```python
from build123d import *

# Parameters (mm, degrees)
BOSS_EXTRUDE1_DEPTH      = 12.7
BOSS_EXTRUDE1_DRAFT      = -1
SKETCH8_W                = 66.675
SKETCH8_H                = 1.5875
CUT_EXTRUDE1_DEPTH       = 139.494635157
CUT_EXTRUDE1_DEPTH_BACK  = 139.494635157
CUT_EXTRUDE3_REACH       = 227.639
CUT_EXTRUDE3_END_RADIUS  = 19.05
SKETCH9_R                = 3.175
BOSS_EXTRUDE2_REACH      = 228.521
BOSS_EXTRUDE2_END_RADIUS = 19.05
BOSS_EXTRUDE2_DRAFT      = 1


with BuildPart() as part:
    # Sketch2 → Boss-Extrude1 (with draft: the straight prism first)
    with BuildSketch(Plane(origin=(0, 0, 0), x_dir=(1, 0, 0), z_dir=(0, 1, 0))):
        with BuildLine():
            Line((-113.50625, 58.7375), (-113.50625, -58.7375))
            ThreePointArc((-113.50625, -58.7375), (-94.45625, -77.7875), (-75.40625, -58.7375))
            Line((-75.40625, -58.7375), (-75.40625, -30.1625))
            Line((-75.40625, -30.1625), (75.40625, -30.1625))
            Line((75.40625, -30.1625), (75.40625, -58.7375))
            ThreePointArc((75.40625, -58.7375), (94.45625, -77.7875), (113.50625, -58.7375))
            Line((113.50625, -58.7375), (113.50625, 58.7375))
            ThreePointArc((113.50625, 58.7375), (94.45625, 77.7875), (75.40625, 58.7375))
            Line((75.40625, 58.7375), (75.40625, 30.1625))
            Line((75.40625, 30.1625), (-75.40625, 30.1625))
            Line((-75.40625, 30.1625), (-75.40625, 58.7375))
            ThreePointArc((-75.40625, 58.7375), (-94.45625, 77.7875), (-113.50625, 58.7375))
        make_face()
        with BuildLine():
            ThreePointArc((-88.9, -63.5), (-94.45625, -69.05625), (-100.0125, -63.5))
            Line((-100.0125, -63.5), (-100.0125, -53.975))
            ThreePointArc((-100.0125, -53.975), (-94.45625, -48.41875), (-88.9, -53.975))
            Line((-88.9, -53.975), (-88.9, -63.5))
        make_face(mode=Mode.SUBTRACT)
        with BuildLine():
            Line((-100.0125, 53.975), (-100.0125, 63.5))
            ThreePointArc((-100.0125, 63.5), (-94.45625, 69.05625), (-88.9, 63.5))
            Line((-88.9, 63.5), (-88.9, 53.975))
            ThreePointArc((-88.9, 53.975), (-94.45625, 48.41875), (-100.0125, 53.975))
        make_face(mode=Mode.SUBTRACT)
        with BuildLine():
            Line((100.0125, 63.5), (100.0125, 53.975))
            ThreePointArc((100.0125, 53.975), (94.45625, 48.41875), (88.9, 53.975))
            Line((88.9, 53.975), (88.9, 63.5))
            ThreePointArc((88.9, 63.5), (94.45625, 69.05625), (100.0125, 63.5))
        make_face(mode=Mode.SUBTRACT)
        with BuildLine():
            Line((100.0125, -53.975), (100.0125, -63.5))
            ThreePointArc((100.0125, -63.5), (94.45625, -69.05625), (88.9, -63.5))
            Line((88.9, -63.5), (88.9, -53.975))
            ThreePointArc((88.9, -53.975), (94.45625, -48.41875), (100.0125, -53.975))
        make_face(mode=Mode.SUBTRACT)
    extrude(amount=BOSS_EXTRUDE1_DEPTH)
    # Boss-Extrude1: the draft: its side faces are tilted about the plane it starts from
    boss_extrude1_sides = [part.faces().sort_by_distance(p)[0] for p in [
        (-113.50625, 6.35, 0),
        (-94.45625, 6.35, 77.7875),
        (-75.40625, 6.35, 44.45),
        (0, 6.35, 30.1625),
        (75.40625, 6.35, 44.45),
        (94.45625, 6.35, 77.7875),
        (113.50625, 6.35, 0),
        (94.45625, 6.35, -77.7875),
        (75.40625, 6.35, -44.45),
        (0, 6.35, -30.1625),
        (-75.40625, 6.35, -44.45),
        (-94.45625, 6.35, -77.7875),
        (-94.45625, 6.35, 48.41875),
        (-88.9, 6.35, 58.7375),
        (-94.45625, 6.35, 69.05625),
        (-100.0125, 6.35, 58.7375),
        (-100.0125, 6.35, -58.7375),
        (-94.45625, 6.35, -69.05625),
        (-88.9, 6.35, -58.7375),
        (-94.45625, 6.35, -48.41875),
        (100.0125, 6.35, -58.7375),
        (94.45625, 6.35, -48.41875),
        (88.9, 6.35, -58.7375),
        (94.45625, 6.35, -69.05625),
        (100.0125, 6.35, 58.7375),
        (94.45625, 6.35, 69.05625),
        (88.9, 6.35, 58.7375),
        (94.45625, 6.35, 48.41875),
    ]]
    draft(boss_extrude1_sides, Plane(origin=(0, 0, 0), x_dir=(1, 0, 0), z_dir=(0, 1, 0)), BOSS_EXTRUDE1_DRAFT)

    # Sketch8 → Cut-Extrude1 (cut, two sides)
    with BuildSketch(Plane.XY) as cut_extrude1_sk:
        with Locations((-33.3375, 11.90625)):
            Rectangle(SKETCH8_W, SKETCH8_H)
        with Locations((33.3375, 11.90625)):
            Rectangle(SKETCH8_W, SKETCH8_H)
    extrude(amount=CUT_EXTRUDE1_DEPTH, mode=Mode.SUBTRACT)
    extrude(cut_extrude1_sk.sketch, amount=-CUT_EXTRUDE1_DEPTH_BACK, mode=Mode.SUBTRACT)



with BuildPart() as body_2:
    # Sketch5 → Revolve2 (revolve)
    with BuildSketch(Plane.XY.offset(9.525), mode=Mode.PRIVATE) as revolve2_sk:
        with BuildLine():
            Line((141.509179325, -122.2375), (141.509179325, -128.5748))
            Line((141.509179325, -128.5748), (136.746679325, -128.5748))
            Line((136.746679325, -128.5748), (136.746679325, -126.20625))
            Line((136.746679325, -126.20625), (82.771679325, -126.20625))
            Line((82.771679325, -126.20625), (82.771679325, -128.5748))
            Line((82.771679325, -128.5748), (78.009179325, -128.5748))
            Line((78.009179325, -128.5748), (78.009179325, -122.2375))
            ThreePointArc((78.009179325, -122.2375), (78.474147309, -121.114967985), (79.596679325, -120.65))
            Line((79.596679325, -120.65), (139.921679325, -120.65))
            ThreePointArc((139.921679325, -120.65), (141.04421134, -121.114967985), (141.509179325, -122.2375))
        make_face()
        with BuildLine():
            Line((-138.684570675, -128.5748), (-138.684570675, -122.2375))
            ThreePointArc((-138.684570675, -122.2375), (-138.219602691, -121.114967985), (-137.097070675, -120.65))
            Line((-137.097070675, -120.65), (-76.772070675, -120.65))
            ThreePointArc((-76.772070675, -120.65), (-75.64953866, -121.114967985), (-75.184570675, -122.2375))
            Line((-75.184570675, -122.2375), (-75.184570675, -128.5748))
            Line((-75.184570675, -128.5748), (-79.947070675, -128.5748))
            Line((-79.947070675, -128.5748), (-79.947070675, -126.20625))
            Line((-79.947070675, -126.20625), (-133.922070675, -126.20625))
            Line((-133.922070675, -126.20625), (-133.922070675, -128.5748))
            Line((-133.922070675, -128.5748), (-138.684570675, -128.5748))
        make_face()
    revolve(revolve2_sk.sketch.rotate(Axis((-113.50625, -139.7, 9.525), (1, 0, 0)), 90), axis=Axis((-113.50625, -139.7, 9.525), (1, 0, 0)))

    # Cut-Extrude3: up to this cylinder (the profile starts inside it)
    cut_extrude3_end = Plane(origin=(1.412304, -139.7, 9.525), z_dir=(-1, 0, 0)) * Cylinder(CUT_EXTRUDE3_END_RADIUS, 717.42175, mode=Mode.PRIVATE)
    # Sketch9 → Cut-Extrude3 (cut, up to the surface)
    with BuildSketch(Plane(origin=(0, -139.7, 9.525), x_dir=(1, 0, 0), z_dir=(0, 0.9396926207859079, 0.3420201433256704)), mode=Mode.PRIVATE) as cut_extrude3_sk1:
        with Locations(Location((-110.109570675, 0, 0), (0, 0, 90))):
            Circle(SKETCH9_R)
    cut_extrude3_tool1 = extrude(cut_extrude3_sk1.sketch, amount=CUT_EXTRUDE3_REACH, mode=Mode.PRIVATE) & cut_extrude3_end
    add(cut_extrude3_tool1.solids().sort_by_distance((-110.109571, -139.7, 9.525))[0], mode=Mode.SUBTRACT)
    # Sketch9 → Cut-Extrude3 (cut, up to the surface)
    with BuildSketch(Plane(origin=(0, -139.7, 9.525), x_dir=(1, 0, 0), z_dir=(0, 0.9396926207859079, 0.3420201433256704)), mode=Mode.PRIVATE) as cut_extrude3_sk2:
        with Locations(Location((112.934179325, 0, 0), (0, 0, 90))):
            Circle(SKETCH9_R)
    cut_extrude3_tool2 = extrude(cut_extrude3_sk2.sketch, amount=CUT_EXTRUDE3_REACH, mode=Mode.PRIVATE) & cut_extrude3_end
    add(cut_extrude3_tool2.solids().sort_by_distance((112.934179, -139.7, 9.525))[0], mode=Mode.SUBTRACT)


with BuildPart() as part_1:
    add(part.part)

    add(body_2.part)  # Boss-Extrude2 merges body 2
    # Boss-Extrude2: up to this cylinder (the profile starts outside it)
    boss_extrude2_end = Plane(origin=(8.945782, -139.7, 9.525), z_dir=(-1, 0, 0)) * Cylinder(BOSS_EXTRUDE2_END_RADIUS, 704.311884, mode=Mode.PRIVATE)



with BuildPart() as boss_extrude2_long_prism_1:
    # Sketch6 → Boss-Extrude2 (the long prism of profile 1, to be tilted and cut off)
    with BuildSketch(Plane(origin=(0, 0, 0), x_dir=(-1, 0, 0), z_dir=(0, -1, 0))):
        Polygon((113.50625, 4.7625), (76.772070675, 4.7625), (76.772070675, -28.575), (86.297070675, -28.575), (86.297070675, -4.7625), (113.50625, -4.7625), align=None)
    extrude(amount=BOSS_EXTRUDE2_REACH)
    boss_extrude2_tool1_sides = [boss_extrude2_long_prism_1.faces().sort_by_distance(p)[0] for p in [
        (-95.139160338, -114.2605, -4.7625),
        (-76.772070675, -114.2605, 11.90625),
        (-81.534570675, -114.2605, 28.575),
        (-86.297070675, -114.2605, 16.66875),
        (-99.901660338, -114.2605, 4.7625),
        (-113.50625, -114.2605, 0),
    ]]
    draft(boss_extrude2_tool1_sides, Plane(origin=(0, 0, 0), x_dir=(-1, 0, 0), z_dir=(0, -1, 0)), BOSS_EXTRUDE2_DRAFT)  # the draft: side faces tilted about the start plane


with BuildPart() as part_2:
    add(part_1.part)
    boss_extrude2_tool1 = boss_extrude2_long_prism_1.part - boss_extrude2_end
    add(boss_extrude2_tool1.solids().sort_by_distance((-95.13916, 0, -4.266437))[0])



with BuildPart() as boss_extrude2_long_prism_2:
    # Sketch6 → Boss-Extrude2 (the long prism of profile 2, to be tilted and cut off)
    with BuildSketch(Plane(origin=(0, 0, 0), x_dir=(-1, 0, 0), z_dir=(0, -1, 0))):
        Polygon((-113.50625, -4.7625), (-113.50625, 4.7625), (-79.596679325, 4.7625), (-79.596679325, -28.575), (-89.121679325, -28.575), (-89.121679325, -4.7625), align=None)
    extrude(amount=BOSS_EXTRUDE2_REACH)
    boss_extrude2_tool2_sides = [boss_extrude2_long_prism_2.faces().sort_by_distance(p)[0] for p in [
        (113.50625, -114.2605, 0),
        (96.551464662, -114.2605, -4.7625),
        (79.596679325, -114.2605, 11.90625),
        (84.359179325, -114.2605, 28.575),
        (89.121679325, -114.2605, 16.66875),
        (101.313964662, -114.2605, 4.7625),
    ]]
    draft(boss_extrude2_tool2_sides, Plane(origin=(0, 0, 0), x_dir=(-1, 0, 0), z_dir=(0, -1, 0)), BOSS_EXTRUDE2_DRAFT)  # the draft: side faces tilted about the start plane


with BuildPart() as part_3:
    add(part_2.part)
    boss_extrude2_tool2 = boss_extrude2_long_prism_2.part - boss_extrude2_end
    add(boss_extrude2_tool2.solids().sort_by_distance((113.030724, 0, 0))[0])


solid = part_3.part
```
The listing builds one solid part. Answer for the finished solid, in the listing's coordinates (mm). Round coordinates to 2 decimals unless told otherwise and drop trailing zeros. Loops run counter-clockwise (first coordinate to the right, second up) from the corner with the lowest first, then second, coordinate; pieces in that order, holes last. Notation, with made-up numbers: (64.5, -19.75) - (104.5, -19.75) arc R26 cw to (104.5, 16.25) - close; hole circle Ø10 at (-1.5, -39). An arc over 180 degrees is marked (long way). Return JSON: item names as keys, results as strings. Group by question number.
1. The part is cut by section D-D on y = -139.7. State how many separate pieces and enclosed holes the cut face has, then the cut area to 3 significant figures.
2. Consider probe 1 along Z at (x, y) = (98.5, -139.7) (3 decimals); probe 2 along X at (y, z) = (-139.5, -2); probe 3 along Z at (x, y) = (-135, -139). Determine where each line is inside the solid, lowest interval first.
3. The mould has two halves that part along X. Classify faces 1 (the flat face through (-138.685, -140, -2)), 2 (the flat face through (-96, 12.7, -1)), 3 (the flat face through (-75.185, -140, 21)): pulls with the +X half, pulls with the -X half, needs draft (parallel to the pull), parting line crosses it, or undercut.
4. The part is cut by section A-A on y = -92.5. Determine the outline of the cut face in (x, z), then the cut area to 3 significant figures.
5. The part is cut by section C-C on y = -74. Determine the outline of the cut face in (x, z), then the cut area to 3 significant figures.
6. The part is cut by section B-B on z = 35.5. Determine the outline of the cut face in (x, y), then the cut area to 3 significant figures.
7. Each of these flat-tipped pins is pushed along its axis until it touches: P1, Ø21.5, axis at y = -137.5, z = 9.5, coming from the -X side; P2, Ø6, axis at y = -112.5, z = 29, coming from the +X side; P3, Ø1, axis at x = -89, y = -110, coming from the +Z side; P4, Ø17.5, axis at y = -140.5, z = 8.5, coming from the -X side. Where does it stop, or does it pass through?
Resolved:
{
 "1": {"separate pieces": "4", "enclosed holes": "0", "area": "1,500 mm²"},
 "2": {"probe 1": "z = -9.525 to -3.969, 23.019 to 28.575", "probe 2": "x = -138.68 to -133.92, -79.95 to -75.18, 78.01 to 82.77, 136.75 to 141.51", "probe 3": "z = -9.51 to -1.58, 20.63 to 28.56"},
 "3": {"face 1": "pulls with the -X half", "face 2": "needs draft", "face 3": "undercut"},
 "4": {"outline": "(-111.89, -3.15) - (-78.39, -3.15) - (-78.39, 26.96) - (-84.68, 26.96) - (-84.68, 3.15) - (-111.89, 3.15) - close; (81.21, -3.15) - (111.89, -3.15) - (111.89, 3.15) - (87.51, 3.15) - (87.51, 26.96) - (81.21, 26.96) - close", "area": "704 mm²"},
 "5": {"outline": "(-112.21, -3.47) - (-78.06, -3.47) - (-78.06, 27.28) - (-85.01, 27.28) - (-85.01, 3.47) - (-112.21, 3.47) - close; (80.89, -3.47) - (112.21, -3.47) - (112.21, 3.47) - (87.83, 3.47) - (87.83, 27.28) - (80.89, 27.28) - close", "area": "785 mm²"},
 "6": {"outline": "(-113.73, 12.7) - (-113.51, 0) - (-75.41, 0) - (-75.18, 12.7) - close; (75.18, 12.7) - (75.41, 0) - (113.51, 0) - (113.73, 12.7) - close", "area": "973 mm²"},
 "7": {"P1": "stops at x = -138.68", "P2": "stops at x = 87.19", "P3": "stops at z = 2.85", "P4": "passes through"}
}
